from build123d import *

# Parameters (mm, degrees)
SKETCH_1_R          = 2.5
EXTRUDE_1_DEPTH     = 8
SKETCH_5_R          = 3
CUT_EXTRUDE_2_DEPTH = 3
SKETCH_7_R          = 2
EXTRUDE_3_DEPTH     = 3
FILLET_5_R          = 2
SKETCH_8_R          = 2.5
CUT_EXTRUDE_3_DEPTH = 3
SKETCH_9_R          = 1.5
EXTRUDE_4_DEPTH     = 4
FILLET_6_R          = 1.5


with BuildPart() as part:
    # 스케치1 → 보스-돌출1 (new body)
    with BuildSketch(Plane.XY):
        with BuildLine():
            Line((-0.451148657, 21.875531488), (-0.451148657, 23.195899803))
            Line((-0.451148657, 23.195899803), (11.359015021, 23.195899803))
            Line((11.359015021, 23.195899803), (11.945796901, 16.807444187))
            Line((11.945796901, 16.807444187), (10.112329073, 13.81338505))
            Line((10.112329073, 13.81338505), (5, 5.464934457))
            Line((5, 5.464934457), (5, 3.83484861))
            Line((5, 3.83484861), (5, 0))
            ThreePointArc((5, 0), (3.535533906, -3.535533906), (0, -5))
            Line((0, -5), (-14.582903299, 0.299385373))
            ThreePointArc((-14.582903299, 0.299385373), (-14.889635684, 0.655255963), (-15, 1.111926907))
            Line((-15, 1.111926907), (-15, 2.937976957))
            Line((-15, 2.937976957), (-9.735777088, 6.555734799))
            ThreePointArc((-9.735777088, 6.555734799), (-9.571850512, 6.512511163), (-9.5, 6.358960817))
            Line((-9.5, 6.358960817), (-9.5, 4.598603361))
            Line((-9.5, 4.598603361), (-7.258120431, 3.851310171))
            Line((-7.258120431, 3.851310171), (-0.451148657, 15.101495802))
            Line((-0.451148657, 15.101495802), (-0.451148657, 21.875531488))
        make_face()
        Circle(SKETCH_1_R, mode=Mode.SUBTRACT)
    extrude(amount=EXTRUDE_1_DEPTH)

    # 스케치5 → 컷-돌출2 (cut)
    with BuildSketch(Plane(origin=(-1.605029546, -4.416736851, 0), x_dir=(0.9398656128397294, -0.34154447704713375, 0), z_dir=(-0.34154447704713375, -0.9398656128397295, 0))):
        with Locations((-9.929236479, 4)):
            Circle(SKETCH_5_R)
    extrude(amount=-CUT_EXTRUDE_2_DEPTH, mode=Mode.SUBTRACT)

    # 스케치7 → 보스-돌출3 (add)
    with BuildSketch(Plane(origin=(-0.580396115, -1.597140012, 0), x_dir=(0.9398656128397294, -0.34154447704713387, 0), z_dir=(-0.34154447704713387, -0.9398656128397294, 0))):
        with Locations((-9.929236479, 4)):
            Circle(SKETCH_7_R)
    extrude(amount=EXTRUDE_3_DEPTH)

    # 필렛5
    fillet_5_edges = [part.edges().sort_by_distance(p)[0] for p in [
        (-12.8169087, -0.342372016, 4),
    ]]
    fillet(fillet_5_edges, radius=FILLET_5_R)

    # 스케치8 → 컷-돌출3 (cut)
    with BuildSketch(Plane(origin=(0, 23.195899803, 0), x_dir=(1, 0, 0), z_dir=(0, 1, 0))):
        with Locations(Location((2.548851343, -4, 0), (0, 0, 270))):
            Circle(SKETCH_8_R)
    extrude(amount=-CUT_EXTRUDE_3_DEPTH, mode=Mode.SUBTRACT)

    # 스케치9 → 보스-돌출4 (add)
    with BuildSketch(Plane(origin=(0, 20.195899803, 0), x_dir=(1, 0, 0), z_dir=(0, 1, 0))):
        with Locations(Location((2.548851343, -4, 0), (0, 0, 270))):
            Circle(SKETCH_9_R)
    extrude(amount=EXTRUDE_4_DEPTH)

    # 필렛6
    fillet_6_edges = [part.edges().sort_by_distance(p)[0] for p in [
        (2.548851343, 24.195899803, 2.5),
    ]]
    fillet(fillet_6_edges, radius=FILLET_6_R)


solid = part.part
Work out the finished part from the listing and answer in its coordinate system (mm). A direction names the side the tool comes from. Round coordinates to 2 decimals unless told otherwise and drop trailing zeros. Write each loop counter-clockwise with the first axis right and the second up, starting at its lowest first coordinate (ties: lowest second). Pieces come first, ordered by that corner, then holes.
1) A tool of negligible diameter and unlimited length cuts with its end or side. For faces 4 (the flat face through (-0.451, 19, 4)), 5 (the flat face through (5, 3, 4)), 6 (the flat face through (11.648, 20.046, 3.944)), 7 (the flat face through (-3.9, 9.4, 3.9)), 8 (the cylindrical face through (1.974, 21.428, 5.386)), from which of +Z, -Z, +X, -X, +Y, -Y can it reach the whole face along a straight path? Write none if from no direction.
2) Given pin 1 Ø4 at (x, y) = (0.5, 20) entering from -Z; pin 2 Ø4.5 at (x, y) = (0, 0) entering from -Z; pin 3 Ø1.5 at (x, z) = (-8, 7) entering from +Y; pin 4 Ø4.5 at (y, z) = (2.5, 4) entering from +X, each flat-ended and moving along its own axis, determine where each tip first touches the part or whether it passes through.
3) A cutting plane is placed at A-A (z = 0.5). Give the vertices of the cut face in (x, y).
4) A cutting plane is placed at D-D (y = 14.5). Give the vertices of the cut face in (x, z).
5) A cutting plane is placed at C-C (x = -6.5). Give the vertices of the cut face in (y, z), plus the area to 3 significant figures.
6) The mould has two halves that part along Z. Classify faces 1 (the flat face through (-15, 2, 4)), 2 (the flat face through (2, 9, 8)), 3 (the cylindrical face through (-9.214, 1.016, 2.226)): pulls with the +Z half, pulls with the -Z half, needs draft (parallel to the pull), parting line crosses it, or undercut.
7) Straight lines are drawn through the part: line 1 (Y direction, x = 0, z = 5.5); line 2 (X direction, y = 21.95, z = 4); line 3 (Y direction, x = -1, z = 3.75). For each, find the intervals that lie inside material, in ascending order.
Completed:
1. face 4: +Z, -Z, -X, +Y
1. face 5: +Z, -Z, +X, -Y
1. face 6: +Z, -Z, +X, +Y
1. face 7: +Z, -Z, +Y
1. face 8: +Y
2. pin 1: stops at z = 0
2. pin 2: passes through
2. pin 3: stops at y = 4.35
2. pin 4: stops at x = 5
3. outline: (-15, 1.11) arc R1 ccw to (-14.58, 0.3) - (0, -5) arc R5 ccw to (5, 0) - (5, 5.46) - (11.95, 16.81) - (11.36, 23.2) - (-0.45, 23.2) - (-0.45, 15.1) - (-7.26, 3.85) - (-9.5, 4.6) - (-9.5, 6.36) arc R0.2 ccw to (-9.74, 6.56) - (-15, 2.94) - close; hole circle Ø5 at (0, 0)
4. outline: (-0.82, 0) - (10.53, 0) - (10.53, 8) - (-0.82, 8) - close
5. outline: (-2.64, 0) - (5.1, 0) - (5.1, 8) - (-2.64, 8) - close
5. area: 61.9 mm2
6. face 1: needs draft
6. face 2: pulls with the +Z half
6. face 3: undercut
7. line 1: y = -5 to -2.5, 2.5 to 23.2
7. line 2: x = -0.45 to 0.05, 1.05 to 4.05, 5.05 to 11.47
7. line 3: y = -4.64 to -2.29, 2.29 to 14.19
